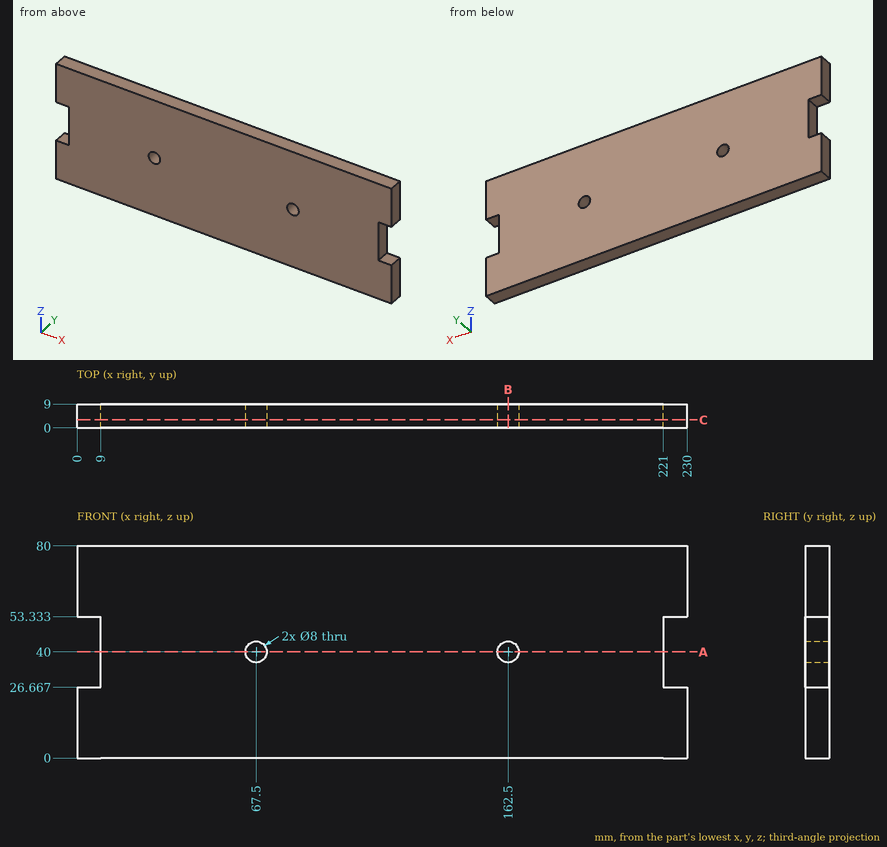
Here's the drawing with two shaded views (mm, measured from the low corner). I have some questions. Give positions to 0.01 mm unless a question says otherwise; leave off trailing zeros. Order: outer loops, then holes, each group sorted by start corner. A loop starts at its lowest first (then second) coordinate and runs counter-clockwise, first axis right, second up.
Q1. Suppose I cut it at C-C, the plane y = 3. Write out the boundary of the cut face in (x, z).
Q2. I'm going to push a flat-ended pin straight in: P1, Ø5, axis at x = 162.5, z = 40, coming from the -Y side. Where does the tip first touch, or does it pass through?
Q3. Suppose I cut it at A-A, the plane z = 40. Write out the boundary of the cut face in (x, y), and give its area (3 significant figures).
Q4. Suppose I cut it at B-B, the plane x = 162.5. Write out the boundary of the cut face in (y, z), and give its area (3 significant figures).
Q5. If I drill on line 1 along X through (y, z) = (4.75, 40); line 2 along X through (y, z) = (1.25, 53); line 3 along Z through (x, y) = (68.5, 2.75), over which ranges is the centre line in solid material (lowest first)?
Solution:
1. outline: (0, 0) - (230, 0) - (230, 26.67) - (221, 26.67) - (221, 53.33) - (230, 53.33) - (230, 80) - (0, 80) - (0, 53.33) - (9, 53.33) - (9, 26.67) - (0, 26.67) - close; hole circle Ø8 at (67.5, 40); hole circle Ø8 at (162.5, 40)
2. P1: passes through
3. outline: (9, 0) - (63.5, 0) - (63.5, 9) - (9, 9) - close; (71.5, 0) - (158.5, 0) - (158.5, 9) - (71.5, 9) - close; (166.5, 0) - (221, 0) - (221, 9) - (166.5, 9) - close
3. area: 1,760 mm2
4. outline: (0, 0) - (9, 0) - (9, 36) - (0, 36) - close; (0, 44) - (9, 44) - (9, 80) - (0, 80) - close
4. area: 648 mm2
5. line 1: x = 9 to 63.5, 71.5 to 158.5, 166.5 to 221
5. line 2: x = 9 to 221
5. line 3: z = 0 to 36.13, 43.87 to 80
